Input: part model. Units: mm. Frame: model coordinates. Face numbers are marked on the shaded views. Give positions to 0.01 mm unless a question says otherwise; leave off trailing zeros. Order: outer loops, then holes, each group sorted by start corner. A loop starts at its lowest first (then second) coordinate and runs counter-clockwise, first axis right, second up. Notation, with made-up numbers: (41, -19) -> (64, -19) arc R15 ccw to (64, 10) -> close; hole circle Ø6 at (55, -11.5). An arc over 180 degrees is marked (long way). Use a Markdown table: item, result. Add a question column.
from build123d import *

# Parameters (mm, degrees)
ESQUISSE1_R        = 1.5
BOSS_EXTRU_1_DEPTH = 5
BOSS_EXTRU_2_DEPTH = 5
CONG_1_R           = 10
CONG_2_R           = 2


with BuildPart() as part:
    # Esquisse1 → Boss.-Extru.1 (new body)
    with BuildSketch(Plane.XY):
        Polygon((0, 0), (37, 0), (37, 18), (12, 18), (12, 55), (0, 55), align=None)
        with Locations((6, 32)):
            Circle(ESQUISSE1_R, mode=Mode.SUBTRACT)
        with Locations((31, 12)):
            Circle(ESQUISSE1_R, mode=Mode.SUBTRACT)
    extrude(amount=BOSS_EXTRU_1_DEPTH)

    # Esquisse2 → Boss.-Extru.2 (add)
    with BuildSketch(Plane.XY.offset(5)):
        Polygon((37, 0), (42, 0), (42, -5), (49.5, -5), (49.5, 0), (64.5, 0), (64.5, -5), (72, -5), (72, 0), (79.5, 0), (79.5, 5), (69, 5), (69, 9), (43, 9), (43, 18), (37, 18), align=None)
        Polygon((0, 0), (-5, 0), (-5, -5), (-12.5, -5), (-12.5, 0), (-32.5, 0), (-32.5, -5), (-40, -5), (-40, 0), (-62.19, 0), (-62.19, 10), (-67.19, 10), (-67.19, 25), (-62.19, 25), (-62.19, 60), (-67.19, 60), (-67.19, 75), (-62.19, 75), (-62.19, 142), (-67.19, 142), (-67.19, 157), (-62.19, 157), (-62.19, 167), (-52.19, 167), (-52.19, 172), (-42.19, 172), (-42.19, 167), (30, 167), (30, 172), (40, 172), (40, 167), (50, 167), (50, 108), (33, 108), (33, 85), (-15, 85), (-15, 55), (0, 55), align=None)
    extrude(amount=-BOSS_EXTRU_2_DEPTH)

    # Congé1
    # the kernel refuses this fillet: 10 mm, written as the material it takes off along each edge
    with BuildSketch(Plane(origin=(43, 18, 29.874685928), x_dir=(0, -1, 0), z_dir=(0, 0, -1))) as cong_1_piece_1:
        with BuildLine():
            CenterArc((10, 9.949874371), CONG_1_R, 180, 84.260829523)
            Line((0, 9.949874371), (-0.2, 9.949874371))
            Line((-0.2, 9.949874371), (-0.2, 0))
            Line((-0.2, 0), (0, -0.2))
            ThreePointArc((0, -0.2), (4.5, -0.2), (8.98, -0.198997487))
            Line((8.98, -0.198997487), (9, 0))
        make_face()
    extrude(amount=54.749371855, mode=Mode.SUBTRACT)

    # Congé2
    cong_2_edges = [part.edges().sort_by_distance(p)[0] for p in [
        (43, 9, 2.5),
    ]]
    fillet(cong_2_edges, radius=CONG_2_R)


solid = part.part
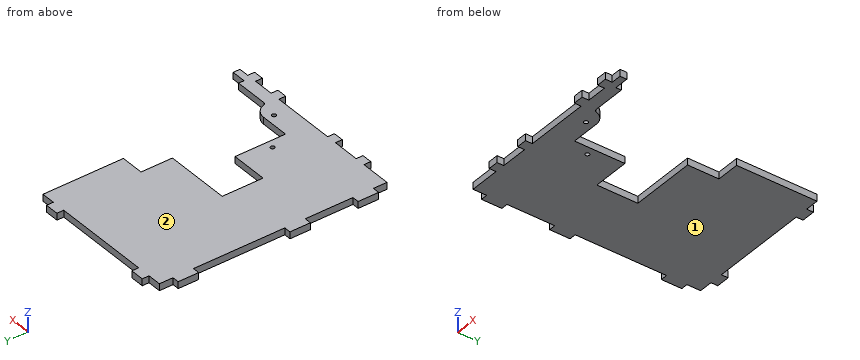
Q1. Section query B-B (y = 88.5). Return loops of the section in (x, z), plus the area to 3 significant figures.
Q2. Ray query, line 1 (Y direction, x = 6, z = 2.55); line 2 (Y direction, x = 31, z = 3.15); line 3 (X direction, y = 145, z = 1.5). Return the intervals inside material, ascending.
Q3. First-contact query: pin 1 (1 mm diameter, centred on y = 120.5, z = 3, fed in from -X); pin 2 (2 mm diameter, centred on x = 5.5, z = 2.5, fed in from +Y); pin 3 (1.8 mm diameter, centred on x = 6, y = 32, fed in from +Z); pin 4 (1.5 mm diameter, centred on x = -63.5, z = 3, fed in from +Y). Flat tips, straight axial feed; report the tip coordinate or a pass-through.
Q4. Section query C-C (x = -50). Return loops of the section in (y, z), plus the area to 3 significant figures.
Q5. Draft query along Z for the marked faces 1 and 2. Return one class per face: +Z half, -Z half, draft (parallel to the pull), parting line (faces both ways), or undercut.
Q6. Section query A-A (z = 1.65). Give the number of separate pieces and of enclosed holes in the cut face, plus the area to 3 significant figures.
Solution:
| question | item | result |
|---|---|---|
| 1 | outline | (-62.19, 0) -> (33, 0) -> (33, 5) -> (-62.19, 5) -> close |
| 1 | area | 476 mm² |
| 2 | line 1 | y = 0 to 30.5, 33.5 to 55, 85 to 167 |
| 2 | line 2 | y = 0 to 10.5, 13.5 to 18, 85 to 172 |
| 2 | line 3 | x = -67.19 to 50 |
| 3 | pin 1 | stops at x = -62.19 |
| 3 | pin 2 | stops at y = 167 |
| 3 | pin 3 | passes through |
| 3 | pin 4 | stops at y = 157 |
| 4 | outline | (0, 0) -> (172, 0) -> (172, 5) -> (0, 5) -> close |
| 4 | area | 860 mm² |
| 5 | face 1 | -Z half |
| 5 | face 2 | +Z half |
| 6 | separate pieces | 1 |
| 6 | enclosed holes | 2 |
| 6 | area | 15,600 mm² |
